```python
from build123d import *

# Parameters (mm, degrees)
BOSS_EXTRUDE1_DEPTH = 3.175
CUT_EXTRUDE1_REACH  = 271.426
SKETCH2_R           = 2.55


with BuildPart() as part:
    # Model → Boss-Extrude1 (new body)
    with BuildSketch(Plane.XY):
        with BuildLine():
            Line((175.500000042, 200), (125.500000042, 200))
            ThreePointArc((125.500000042, 200), (121.964466136, 198.535533906), (120.500000042, 195))
            Line((120.500000042, 195), (120.500000042, 177.5))
            ThreePointArc((120.500000042, 177.5), (119.035533948, 173.964466094), (115.500000042, 172.5))
            Line((115.500000042, 172.5), (-115.500000042, 172.5))
            ThreePointArc((-115.500000042, 172.5), (-119.035533948, 173.964466094), (-120.500000042, 177.5))
            Line((-120.500000042, 177.5), (-120.500000042, 195))
            ThreePointArc((-120.500000042, 195), (-121.964466136, 198.535533906), (-125.500000042, 200))
            Line((-125.500000042, 200), (-175.500000042, 200))
            ThreePointArc((-175.500000042, 200), (-179.035533948, 198.535533906), (-180.500000042, 195))
            Line((-180.500000042, 195), (-180.500000042, -195))
            ThreePointArc((-180.500000042, -195), (-179.035533948, -198.535533906), (-175.500000042, -200))
            Line((-175.500000042, -200), (-125.500000042, -200))
            ThreePointArc((-125.500000042, -200), (-121.964466136, -198.535533906), (-120.500000042, -195))
            Line((-120.500000042, -195), (-120.500000042, -177.5))
            ThreePointArc((-120.500000042, -177.5), (-119.035533948, -173.964466094), (-115.500000042, -172.5))
            Line((-115.500000042, -172.5), (115.500000042, -172.5))
            ThreePointArc((115.500000042, -172.5), (119.035533948, -173.964466094), (120.500000042, -177.5))
            Line((120.500000042, -177.5), (120.500000042, -195))
            ThreePointArc((120.500000042, -195), (121.964466136, -198.535533906), (125.500000042, -200))
            Line((125.500000042, -200), (175.500000042, -200))
            ThreePointArc((175.500000042, -200), (179.035533948, -198.535533906), (180.500000042, -195))
            Line((180.500000042, -195), (180.500000042, 195))
            ThreePointArc((180.500000042, 195), (179.035533948, 198.535533906), (175.500000042, 200))
        make_face()
    extrude(amount=BOSS_EXTRUDE1_DEPTH)

    # Sketch2 → Cut-Extrude1 (cut, up to next)
    with BuildSketch(Plane.XY.offset(3.175), mode=Mode.PRIVATE) as cut_extrude1_sk1:
        with Locations((-150.5, 190.5)):
            Circle(SKETCH2_R)
    cut_extrude1_tool1 = extrude(cut_extrude1_sk1.sketch, amount=-CUT_EXTRUDE1_REACH, mode=Mode.PRIVATE) & part.part
    # Sketch2 → Cut-Extrude1 (cut, up to next)
    with BuildSketch(Plane.XY.offset(3.175), mode=Mode.PRIVATE) as cut_extrude1_sk2:
        with Locations((-150.5, -190.5)):
            Circle(SKETCH2_R)
    cut_extrude1_tool2 = extrude(cut_extrude1_sk2.sketch, amount=-CUT_EXTRUDE1_REACH, mode=Mode.PRIVATE) & part.part
    # Sketch2 → Cut-Extrude1 (cut, up to next)
    with BuildSketch(Plane.XY.offset(3.175), mode=Mode.PRIVATE) as cut_extrude1_sk3:
        with Locations((150.5, -190.5)):
            Circle(SKETCH2_R)
    cut_extrude1_tool3 = extrude(cut_extrude1_sk3.sketch, amount=-CUT_EXTRUDE1_REACH, mode=Mode.PRIVATE) & part.part
    # Sketch2 → Cut-Extrude1 (cut, up to next)
    with BuildSketch(Plane.XY.offset(3.175), mode=Mode.PRIVATE) as cut_extrude1_sk4:
        with Locations((150.5, 190.5)):
            Circle(SKETCH2_R)
    cut_extrude1_tool4 = extrude(cut_extrude1_sk4.sketch, amount=-CUT_EXTRUDE1_REACH, mode=Mode.PRIVATE) & part.part
    add(cut_extrude1_tool1.solids().sort_by_distance((-150.5, 190.5, 3.175))[0], mode=Mode.SUBTRACT)
    add(cut_extrude1_tool2.solids().sort_by_distance((-150.5, -190.5, 3.175))[0], mode=Mode.SUBTRACT)
    add(cut_extrude1_tool3.solids().sort_by_distance((150.5, -190.5, 3.175))[0], mode=Mode.SUBTRACT)
    add(cut_extrude1_tool4.solids().sort_by_distance((150.5, 190.5, 3.175))[0], mode=Mode.SUBTRACT)


solid = part.part
```
Can you work these out from the model? Positions are in its coordinate system, mm. Round coordinates to 2 decimals unless told otherwise and drop trailing zeros. Loops run counter-clockwise (first coordinate to the right, second up) from the corner with the lowest first, then second, coordinate; pieces in that order, holes last. Notation, with made-up numbers: M -39,68 L -17,68 A28 cw -17,103 Z; hole C 57.5,-26.5 d1. An arc over 180 degrees is marked long. Answer as a JSON object with one key per item and string values. Group by question number.
Q1. Will this pin go through, and if not, where does the flat tip stop? pin 1 (1.5 mm diameter, centred on x = 32.5, z = 1.5, fed in from -Y).
Q2. Imagine slicing it at A-A, the plane z = 1.6. Please give me the cut outline in (x, y).
Q3. Imagine slicing it at B-B, the plane x = 19. Please give me the cut outline in (y, z) (3 decimals), then the cut area to 3 significant figures.
Q4. Please list where these lines run through material, in increasing order: L1, parallel to X at y = -190.5, z = 2; L2, parallel to Y at x = -150.5, z = 0.7; L3, parallel to Y at x = -87.5, z = 1.9.
Findings:
{
 "1": {"pin 1": "stops at y = -172.5"},
 "2": {"outline": "M -180.5,-195 A5 ccw -175.5,-200 L -125.5,-200 A5 ccw -120.5,-195 L -120.5,-177.5 A5 cw -115.5,-172.5 L 115.5,-172.5 A5 cw 120.5,-177.5 L 120.5,-195 A5 ccw 125.5,-200 L 175.5,-200 A5 ccw 180.5,-195 L 180.5,195 A5 ccw 175.5,200 L 125.5,200 A5 ccw 120.5,195 L 120.5,177.5 A5 cw 115.5,172.5 L -115.5,172.5 A5 cw -120.5,177.5 L -120.5,195 A5 ccw -125.5,200 L -175.5,200 A5 ccw -180.5,195 Z; hole C -150.5,-190.5 d5.1; hole C -150.5,190.5 d5.1; hole C 150.5,-190.5 d5.1; hole C 150.5,190.5 d5.1"},
 "3": {"outline": "M -172.5,0 L 172.5,0 L 172.5,3.175 L -172.5,3.175 Z", "area": "1,100 mm2"},
 "4": {"L1": "x = -180.5 to -153.05, -147.95 to -120.5, 120.5 to 147.95, 153.05 to 180.5", "L2": "y = -200 to -193.05, -187.95 to 187.95, 193.05 to 200", "L3": "y = -172.5 to 172.5"}
}
